from build123d import *

# Parameters (mm, degrees)
SKETCH1_R                = 50.8
BOSS_EXTRUDE1_DEPTH      = 686.4
BOSS_EXTRUDE1_DEPTH_BACK = 1363.6
SKETCH2_R                = 450
BOSS_EXTRUDE2_DEPTH      = 12.7
SKETCH3_R                = 222.25
BOSS_EXTRUDE3_DEPTH      = 1200


with BuildPart() as part:
    # Sketch1 → Boss-Extrude1 (new body, two sides)
    with BuildSketch(Plane.XY) as boss_extrude1_sk:
        Circle(SKETCH1_R)
    extrude(amount=BOSS_EXTRUDE1_DEPTH)
    extrude(boss_extrude1_sk.sketch, amount=-BOSS_EXTRUDE1_DEPTH_BACK)

    # Sketch2 → Boss-Extrude2 (add)
    with BuildSketch(Plane.XY.offset(-1363.6)):
        Circle(SKETCH2_R)
    extrude(amount=BOSS_EXTRUDE2_DEPTH)

    # Sketch3 → Boss-Extrude3 (add)
    with BuildSketch(Plane.XY.offset(-1350.9)):
        Circle(SKETCH3_R)
    extrude(amount=BOSS_EXTRUDE3_DEPTH)


solid = part.part
Work out the finished part from the listing and answer in its coordinate system (mm). A direction names the side the tool comes from. Coordinates: 2 decimals unless noted, no trailing zeros. Loops run counter-clockwise (first coordinate to the right, second up) from the corner with the lowest first, then second, coordinate; pieces in that order, holes last. Notation, with made-up numbers: (-35.75, 0) -> (-25.75, 0) arc R14 ccw to (-25.75, 10) -> close; hole circle Ø6 at (-25.75, -17.75). An arc over 180 degrees is marked (long way). Write each question's results on one line, items separated by ' | '. Start each with the question number.
1) For faces 3 (the cylindrical face through (-28.93, 220.36, -759.3)), 4 (the flat face through (-1, 1, 686.4)), determine the directions among +Z, -Z, +X, -X, +Y, -Y from which every point of the face is accessible in a straight line to the end or side of a thin tool.
2) Find section C-C on z = -1165. Determine the outline of the cut face in (x, y), then the cut area to 3 significant figures.
3) Find section A-A on x = 0. Determine the outline of the cut face in (y, z), then the cut area to 3 significant figures.
4) Flat-ended cylindrical pins translate along their axes: P1, Ø10, axis at y = 112.5, z = -449, coming from the +X side; P2, Ø5, axis at x = 150.5, z = -813.5, coming from the -Y side; P3, Ø4, axis at y = 200, z = -594, coming from the -X side. Find the tip coordinate at first contact, or state that the pin passes through.
5) The mould has two halves that part along X. Classify faces 1 (the cylindrical face through (-11.012, -49.592, 273.611)), 2 (the flat face through (-53, 3, -150.9)): pulls with the +X half, pulls with the -X half, needs draft (parallel to the pull), parting line crosses it, or undercut.
6) Find section D-D on y = -165.5. Determine the outline of the cut face in (x, z).
7) Consider line 1 along Z through (x, y) = (19.5, 156.5); line 2 along Z through (x, y) = (-253.5, -191); line 3 along X through (y, z) = (58.5, -986). Determine where each line is inside the solid, lowest interval first.
Response values:
1) face 3: +Z | face 4: +Z, +X, -X, +Y, -Y
2) outline: circle Ø444.5 at (0, 0) | area: 155,000 mm^2
3) outline: (-450, -1363.6) -> (450, -1363.6) -> (450, -1350.9) -> (222.25, -1350.9) -> (222.25, -150.9) -> (50.8, -150.9) -> (50.8, 686.4) -> (-50.8, 686.4) -> (-50.8, -150.9) -> (-222.25, -150.9) -> (-222.25, -1350.9) -> (-450, -1350.9) -> close | area: 630,000 mm^2
4) P1: stops at x = 194.52 | P2: stops at y = -165.8 | P3: stops at x = -100.95
5) face 1: parting line crosses it | face 2: needs draft
6) outline: (-418.46, -1363.6) -> (418.46, -1363.6) -> (418.46, -1350.9) -> (148.34, -1350.9) -> (148.34, -150.9) -> (-148.34, -150.9) -> (-148.34, -1350.9) -> (-418.46, -1350.9) -> close
7) line 1: z = -1363.6 to -150.9 | line 2: z = -1363.6 to -1350.9 | line 3: x = -214.41 to 214.41
